Geometry: final body of the model. Coordinates: model frame, mm. A direction names the side the tool comes from. Coordinates: 2 decimals unless noted, no trailing zeros. Loops run counter-clockwise (first coordinate to the right, second up) from the corner with the lowest first, then second, coordinate; pieces in that order, holes last. Notation, with made-up numbers: (44, 70) - (100, 70) arc R22 cw to (100, 78) - close; hole circle Ø3 at (-40, 49.25). An arc over 180 degrees is marked (long way). Answer in a Markdown table with one row per item.
from build123d import *

# Parameters (mm, degrees)
F1_DEPTH = 155.702
F3_DEPTH = 25.4


with BuildPart() as f1:
    # F0 (on Top) → F1 (new body)
    with BuildSketch(Plane.XY):
        Polygon((-35.026107, 29.188428), (-51.641054, 30.086534), (-51.641054, -25.595998), (24.6979, -25.595998), (24.6979, 29.188428), (15.267792, 29.188428), (15.267792, -16.614946), (-35.026107, -16.614946), align=None)
    extrude(amount=F1_DEPTH)

    # F2 (on face) → F3 (join)
    with BuildSketch(Plane(origin=(15.267792, 0, 0), x_dir=(0, -1, 0), z_dir=(-1, 0, 0))):
        Polygon((0, 139.685988), (-13.539952, 120.63428), (-3.559254, 114.443869), (9.554391, 132.895732), align=None)
    extrude(amount=F3_DEPTH)


solid = f1.part
(1) Ray query, probe 1 along X at (y, z) = (20, 92); probe 2 along Y at (x, z) = (8, 90); probe 3 along Y at (x, z) = (20.5, 145.5). Return the intervals inside material, ascending.
Verdict:
| item | result |
|---|---|
| probe 1 | x = -51.64 to -35.03, 15.27 to 24.7 |
| probe 2 | y = -25.6 to -16.61 |
| probe 3 | y = -25.6 to 29.19 |
(2) Cut plane B-B on y = 19. Output: boundary loops of the cut face in (x, z), then the cut area to 3 significant figures.
Verdict:
| item | result |
|---|---|
| outline | (-51.64, 0) - (-35.03, 0) - (-35.03, 155.7) - (-51.64, 155.7) - close; (15.27, 0) - (24.7, 0) - (24.7, 155.7) - (15.27, 155.7) - close |
| area | 4,060 mm² |
(3) Pull-direction query (X, two-part tool) for faces 6 (the face through (2.746, 8.619, 117.582)), 7 (the face through (-43.22, 29.63, 76.76)), 8 (the face through (-14, -25.596, 77)); classes: pulls with the +X half, pulls with the -X half, needs draft (parallel to the pull), parting line crosses it, or undercut.
Verdict:
| item | result |
|---|---|
| face 6 | undercut |
| face 7 | pulls with the +X half |
| face 8 | needs draft |
(4) Cut plane C-C on z = 82. Output: boundary loops of the cut face in (x, y), then the cut area to 3 significant figures.
Verdict:
| item | result |
|---|---|
| outline | (-51.64, -25.6) - (24.7, -25.6) - (24.7, 29.19) - (15.27, 29.19) - (15.27, -16.61) - (-35.03, -16.61) - (-35.03, 29.19) - (-51.64, 30.09) - close |
| area | 1,890 mm² |
(5) First-contact query: pin 1 Ø10 at (x, y) = (-6.5, -7) entering from +Z; pin 2 Ø25 at (x, z) = (-11.5, 82.5) entering from +Y; pin 3 Ø5 at (x, z) = (-33, 124) entering from +Y. Flat tips, straight axial feed; report the tip coordinate or a pass-through.
Verdict:
| item | result |
|---|---|
| pin 1 | stops at z = 138.26 |
| pin 2 | stops at y = -16.61 |
| pin 3 | stops at y = 29.21 |
(6) Cut plane D-D on y = -4.5. Output: boundary loops of the cut face in (x, z).
Verdict:
| item | result |
|---|---|
| outline | (-51.64, 0) - (-35.03, 0) - (-35.03, 155.7) - (-51.64, 155.7) - close; (-10.13, 125.78) - (15.27, 125.78) - (15.27, 0) - (24.7, 0) - (24.7, 155.7) - (15.27, 155.7) - (15.27, 136.49) - (-10.13, 136.49) - close |
(7) Access query for faces 1 (the face through (2.746, -4.844, 136.243)), 2 (the face through (20, 29.188, 77)), 3 (the face through (2.75, 6.68, 130.29)), 4 (the face through (-35.026, 6, 77)), 5 (the face through (2.746, -2.906, 123.541)). Directions: +Z, -Z, +X, -X, +Y, -Y. A direction counts if a zero-diameter tool reaches every point of the face in a straight line with its end or side. Return the directions, or none.
Verdict:
| item | result |
|---|---|
| face 1 | +Z |
| face 2 | +Z, -Z, +X, +Y |
| face 3 | +Z, +Y |
| face 4 | +Z, -Z, +Y |
| face 5 | -Z |
(8) Cut plane A-A on x = 4.5. Output: boundary loops of the cut face in (y, z).
Verdict:
| item | result |
|---|---|
| outline | (-25.6, 0) - (-16.61, 0) - (-16.61, 155.7) - (-25.6, 155.7) - close; (-9.55, 132.9) - (3.56, 114.44) - (13.54, 120.63) - (0, 139.69) - close |
